from build123d import *

# Parameters (mm, degrees)
F1_DEPTH = 90
F2_R     = 6
F3_DEPTH = 20.001


with BuildPart() as f1:
    # F0 (on Top) → F1 (new body)
    with BuildSketch(Plane.XY):
        Polygon((-70, 10), (-70, 0), (-30, 0), (-30, 10), (25, 10), (25, 0), (65, 0), (65, 10), (35, 10), (35, 20), (-40, 20), (-40, 10), align=None)
    extrude(amount=F1_DEPTH)

    # F2 (on Front) → F3 (cut, through all)
    with BuildSketch(Plane.XZ):
        with Locations((-55, 20)):
            Circle(F2_R)
        with Locations((-55, 70)):
            Circle(F2_R)
        with Locations((50, 70)):
            Circle(F2_R)
        with Locations((50, 20)):
            Circle(F2_R)
    extrude(amount=-F3_DEPTH, mode=Mode.SUBTRACT)


solid = f1.part
For this review, take the finished solid that the model builds, in its own axes (mm). A direction names the side the tool comes from. Round coordinates to 2 decimals unless told otherwise and drop trailing zeros. Order: outer loops, then holes, each group sorted by start corner. A loop starts at its lowest first (then second) coordinate and runs counter-clockwise, first axis right, second up. Notation, with made-up numbers: M 19,1.25 L 28,1.25 A15 ccw 28,19.25 Z; hole C 43,40.5 d3. An arc over 180 degrees is marked long. Use a Markdown table: item, result. Add a question column.
Item 1: Add section B-B, the plane x = -55. Give the boundary of the cut face in (y, z), then the cut area to 3 significant figures.
Item 2: Add section A-A, the plane z = 70. Give the boundary of the cut face in (x, y), then the cut area to 3 significant figures.
Item 3: Add section D-D, the plane y = 14.5. Give the boundary of the cut face in (x, z), then the cut area to 3 significant figures.
Item 4: Mouldability with a two-part tool opening along Z and no side actions: class faces 6 (the cylindrical face through (-61, 5, 20)), 7 (the flat face through (-70, 5, 44)), 8 (the flat face through (-3, 12, 90)) as released by +Z, released by -Z, zero draft, split by the parting line, or undercut.
Item 5: Tool access review of faces 1 (the flat face through (-3, 10, 44)), 2 (the flat face through (-2, 20, 44)), 3 (the flat face through (-55, 10, 44)), 4 (the flat face through (65, 5, 44)), 5 (the flat face through (35, 15, 44)): name each direction out of +Z, -Z, +X, -X, +Y, -Y from which nothing blocks a thin tool from reaching the whole face with its end or side.
Item 6: To check wall thickness, follow line 1 along Z through (x, y) = (-55, 2.25); line 2 along X through (y, z) = (2.5, 48); line 3 along Z through (x, y) = (55, 9.5). State the ranges of each line that lie inside material, in increasing order.
Item 7: Add section C-C, the plane z = 50.5. Give the boundary of the cut face in (x, y), then the cut area to 3 significant figures.
Item 8: Insertion check: pin 1 (1.5 mm diameter, centred on x = 40.5, z = 40, fed in from +Y); pin 2 (5 mm diameter, centred on x = 3, z = 68.5, fed in from -Y); pin 3 (5 mm diameter, centred on y = 15, z = 33, fed in from -X). Each pin has a flat end and moves straight along its axis. Give the tip position at first contact, or say it passes through.
Geometry results:
| question | item | result |
|---|---|---|
| 1 | outline | M 0,0 L 10,0 L 10,14 L 0,14 Z; M 0,26 L 10,26 L 10,64 L 0,64 Z; M 0,76 L 10,76 L 10,90 L 0,90 Z |
| 1 | area | 660 mm² |
| 2 | outline | M -70,0 L -61,0 L -61,10 L -70,10 Z; M -49,0 L -30,0 L -30,10 L 25,10 L 25,0 L 44,0 L 44,10 L 35,10 L 35,20 L -40,20 L -40,10 L -49,10 Z; M 56,0 L 65,0 L 65,10 L 56,10 Z |
| 2 | area | 1,310 mm² |
| 3 | outline | M -40,0 L 35,0 L 35,90 L -40,90 Z |
| 3 | area | 6,750 mm² |
| 4 | face 6 | undercut |
| 4 | face 7 | zero draft |
| 4 | face 8 | released by +Z |
| 5 | face 1 | +Z, -Z, -Y |
| 5 | face 2 | +Z, -Z, +X, -X, +Y |
| 5 | face 3 | +Z, -Z, -X, +Y |
| 5 | face 4 | +Z, -Z, +X, +Y, -Y |
| 5 | face 5 | +Z, -Z, +X, +Y |
| 6 | line 1 | z = 0 to 14, 26 to 64, 76 to 90 |
| 6 | line 2 | x = -70 to -30, 25 to 65 |
| 6 | line 3 | z = 0 to 16.68, 23.32 to 66.68, 73.32 to 90 |
| 7 | outline | M -70,0 L -30,0 L -30,10 L 25,10 L 25,0 L 65,0 L 65,10 L 35,10 L 35,20 L -40,20 L -40,10 L -70,10 Z |
| 7 | area | 1,550 mm² |
| 8 | pin 1 | stops at y = 10 |
| 8 | pin 2 | stops at y = 10 |
| 8 | pin 3 | stops at x = -40 |
